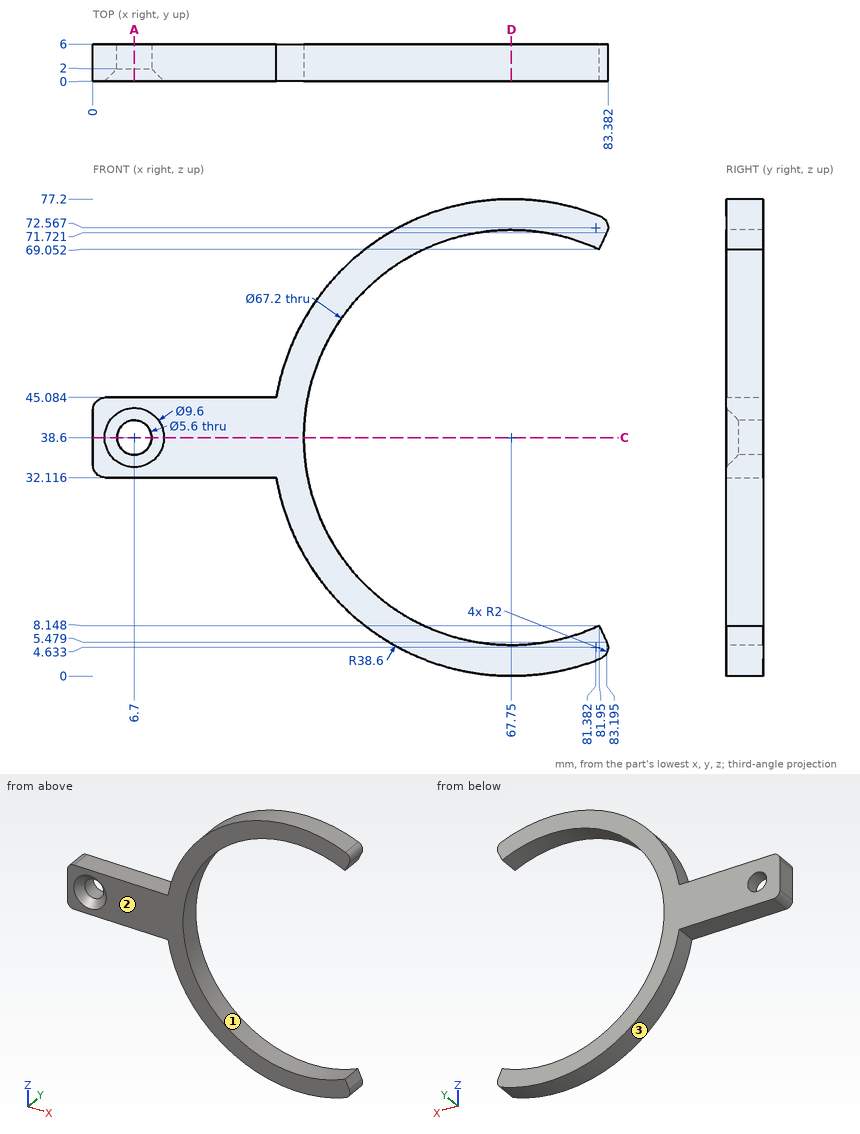
Study the drawing (mm; zero at the part's minimum x, y, z) and answer. Round coordinates to 2 decimals unless told otherwise and drop trailing zeros. Loops run counter-clockwise (first coordinate to the right, second up) from the corner with the lowest first, then second, coordinate; pieces in that order, holes last.
Q1. Section D-D, the plane x = 67.75 is taken. Determine the outline of the cut face in (y, z), then the cut area to 3 significant figures.
Q2. For a pull along Z with two mould halves and no side action, classify the marked faces 1, 2 and 3 as released by +Z, released by -Z, zero draft, split by the parting line, or undercut.
Q3. Section C-C, the plane z = 38.6 is taken. Determine the outline of the cut face in (x, y), then the cut area to 3 significant figures.
Q4. Find the intervals of material crossed by line 1 (Z direction, x = 6.7, y = 3.8) (1 decimal); line 2 (Z direction, x = 67.75, y = 3.5); line 3 (X direction, y = 3.85, z = 38.6), in increasing order.
Q5. Section A-A, the plane x = 6.7 is taken. Determine the outline of the cut face in (y, z) (1 decimal), then the cut area to 3 significant figures.
Q6. Given pin 1 Ø1 at (y, z) = (4.5, 32.5) entering from +X (1 decimal); pin 2 Ø1 at (x, y) = (11, 4) entering from +Z; pin 3 Ø3 at (x, y) = (46, 3.5) entering from +Z; pin 4 Ø10 at (x, z) = (39, 17.5) entering from -Y, each flat-ended and moving along its own axis, determine where each tip first touches the part or whether it passes through.
Completed:
1. outline: (0, 0) - (6, 0) - (6, 5) - (0, 5) - close; (0, 72.2) - (6, 72.2) - (6, 77.2) - (0, 77.2) - close
1. area: 60.0 mm2
2. face 1: undercut
2. face 2: zero draft
2. face 3: released by -Z
3. outline: (0, 0) - (1.9, 0) - (3.9, 2) - (3.9, 6) - (0, 6) - close; (9.5, 2) - (11.5, 0) - (34.15, 0) - (34.15, 6) - (9.5, 6) - close
3. area: 167 mm2
4. line 1: z = 32.1 to 35.8, 41.4 to 45.1
4. line 2: z = 0 to 5, 72.2 to 77.2
4. line 3: x = 0 to 3.9, 9.5 to 34.15
5. outline: (0, 32.1) - (6, 32.1) - (6, 35.8) - (2, 35.8) - (0, 33.8) - close; (0, 43.4) - (2, 41.4) - (6, 41.4) - (6, 45.1) - (0, 45.1) - close
5. area: 40.2 mm2
6. pin 1: stops at x = 34.8
6. pin 2: stops at z = 45.08
6. pin 3: stops at z = 71.46
6. pin 4: stops at y = 0
